Design review of the part shown in the three views and the two pictorial views. Dimensions are in mm from the part's minimum x, y and z. A direction names the side the tool comes from. Give positions to 0.01 mm unless a question says otherwise; leave off trailing zeros. Loops run counter-clockwise (first coordinate to the right, second up) from the corner with the lowest first, then second, coordinate; pieces in that order, holes last. Notation, with made-up numbers: (76, 6.25) -> (100, 6.25) arc R23 ccw to (100, 29.25) -> close; hole circle Ø3 at (76, 4). An arc over 180 degrees is marked (long way). Answer as CSV lines item,"result".
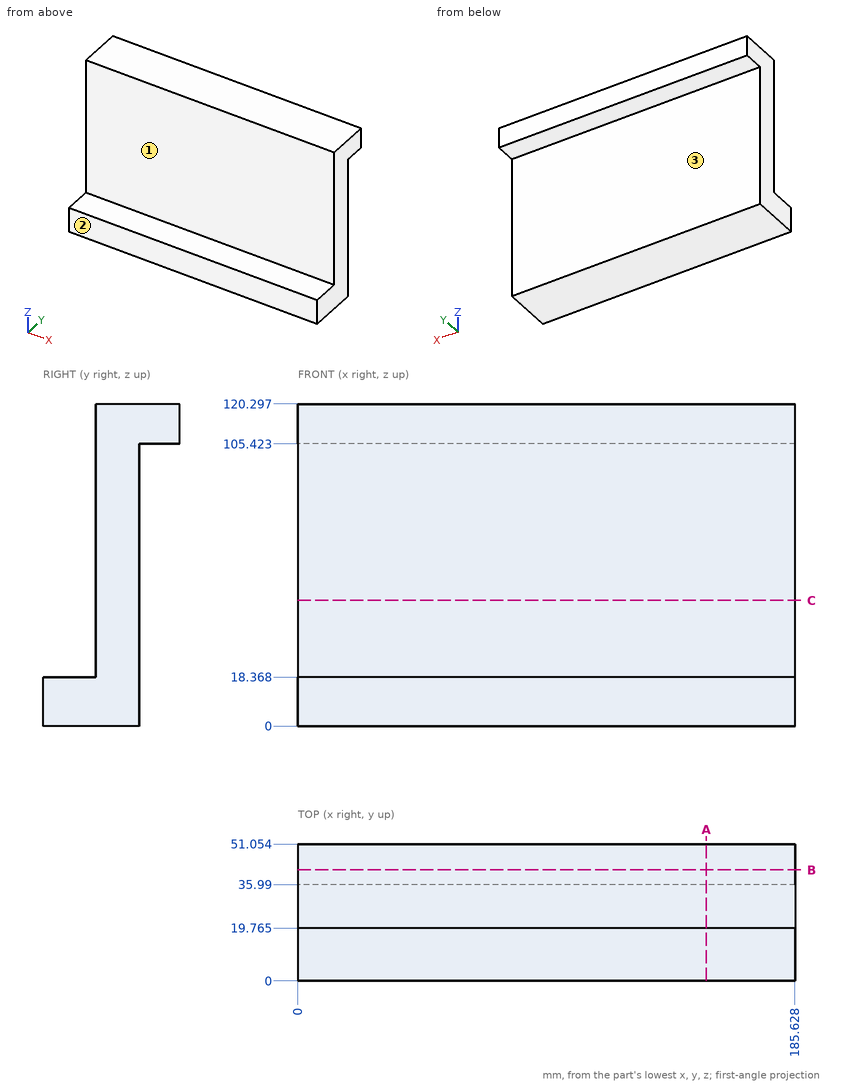
Q1. Clearance check with flat-ended pins moving along their axes: pin 1 Ø10 at (x, y) = (137.5, 14) entering from +Z; pin 2 Ø12 at (y, z) = (40, 92.5) entering from -X; pin 3 Ø16.5 at (x, y) = (80.5, 45.5) entering from -Z. State where each tip first meets the part, or that it passes through.
Filled sheet:
pin 1,"stops at z = 18.37"
pin 2,"stops at x = 0"
pin 3,"stops at z = 105.42"
Q2. To check wall thickness, follow probe 1 along Z at (x, y) = (159.5, 6.5); probe 2 along Y at (x, z) = (34, 10); probe 3 along Z at (x, y) = (21.5, 41). State the ranges of each line that lie inside material, in increasing order. Write a range as from..to.
Filled sheet:
probe 1,"z = 0..18.37"
probe 2,"y = 0..35.99"
probe 3,"z = 105.42..120.3"
Q3. We need section C-C, the plane z = 47. State the section outline as (x, y) points (1 decimal), and give its area (3 significant figures).
Filled sheet:
outline,"(0, 19.8) -> (185.6, 19.8) -> (185.6, 36) -> (0, 36) -> close"
area,"3,010 mm^2"
Q4. We need section A-A, the plane x = 152.5. State the section outline as (y, z) points (1 decimal).
Filled sheet:
outline,"(0, 0) -> (36, 0) -> (36, 105.4) -> (51.1, 105.4) -> (51.1, 120.3) -> (19.8, 120.3) -> (19.8, 18.4) -> (0, 18.4) -> close"
Q5. For the marked faces 1, 2 and 3, list the 3-axis set-ups (+Z, -Z, +X, -X, +Y, -Y) from which the entire face can be reached by the end or side of a thin tool; tool diameter is ignored.
Filled sheet:
face 1,"+Z, +X, -X, -Y"
face 2,"+Z, -Z, +X, -X, -Y"
face 3,"-Z, +X, -X, +Y"
Q6. We need section B-B, the plane y = 41.5. State the section outline as (x, z) points, and give its area (3 significant figures).
Filled sheet:
outline,"(0, 105.42) -> (185.63, 105.42) -> (185.63, 120.3) -> (0, 120.3) -> close"
area,"2,760 mm^2"
